```python
from build123d import *

# Parameters (mm, degrees)
F0_W            = 31.75
F0_H            = 6.35
F0_W_2          = 12.7
F0_H_2          = 101.6
F1_DEPTH        = 6.35
F2_DEPTH        = 76.2
F3_W            = 12.7
F3_H            = 68.58
F4_DEPTH        = 6.35
F5_W            = 12.7
F5_H            = 22.225
F6_DEPTH        = 6.35
F7_D            = 1.5875
F7_CSINK_D      = 3.175
F7_CSINK_ANGLE  = 90
F8_R            = 6.34999
F10_D           = 3.175
F12_D           = 3.175
F12_CSINK_D     = 6.35
F12_CSINK_ANGLE = 90
F13_R           = 1.5875
F14_DEPTH       = 12.7


# Not quite as in the source:
# - a fillet or chamfer is up to 0.001 mm smaller than in the source, because OpenCascade refuses the exact size


with BuildPart() as f1:
    # F0 (on Front) → F1 (new body)
    with BuildSketch(Plane.XZ):
        with Locations((-22.225, 174.625)):
            Rectangle(F0_W, F0_H)
        with Locations((22.225, 174.625)):
            Rectangle(F0_W, F0_H)
        with Locations((-22.225, 3.175)):
            Rectangle(F0_W, F0_H)
        with Locations((22.225, 3.175)):
            Rectangle(F0_W, F0_H)
        Polygon((-6.35, 171.45), (-38.1, 171.45), (-38.1, 108.712), (-31.75, 108.712), (-31.75, 69.088), (-38.1, 69.088), (-38.1, 6.35), (-6.35, 6.35), (-6.35, 22.225), (6.35, 22.225), (6.35, 6.35), (38.1, 6.35), (38.1, 69.088), (31.75, 69.088), (31.75, 108.712), (38.1, 108.712), (38.1, 171.45), (6.35, 171.45), (6.35, 161.925), (-6.35, 161.925), align=None)
        with Locations((0, 92.075)):
            Rectangle(F0_W_2, F0_H_2, mode=Mode.SUBTRACT)
    extrude(amount=F1_DEPTH)

    # F0 (on Front) → F2 (join)
    with BuildSketch(Plane.XZ):
        with Locations((-22.225, 174.625)):
            Rectangle(F0_W, F0_H)
        with Locations((22.225, 174.625)):
            Rectangle(F0_W, F0_H)
        with Locations((-22.225, 3.175)):
            Rectangle(F0_W, F0_H)
        with Locations((22.225, 3.175)):
            Rectangle(F0_W, F0_H)
        with Locations((0, 3.175)):
            Rectangle(F0_W_2, F0_H)
        with Locations((0, 174.625)):
            Rectangle(F0_W_2, F0_H)
    extrude(amount=F2_DEPTH)

    # F3 (on face) → F4 (cut, through all)
    with BuildSketch(Plane.XY.offset(177.8)):
        with Locations((0, -34.29)):
            Rectangle(F3_W, F3_H)
    extrude(amount=-F4_DEPTH, mode=Mode.SUBTRACT)

    # F5 (on face) → F6 (cut, through all)
    with BuildSketch(Plane(origin=(0, 0, 0), x_dir=(1, 0, 0), z_dir=(0, 0, -1))):
        with Locations((0, 11.1125)):
            Rectangle(F5_W, F5_H)
    extrude(amount=-F6_DEPTH, mode=Mode.SUBTRACT)

    # F7 (through all)
    with Locations(Plane(origin=(0, 0, 0), x_dir=(1, 0, 0), z_dir=(0, 1, 0))):
        with Locations((-3.175, -158.75), (3.175, -158.75)):
            CounterSinkHole(F7_D / 2, F7_CSINK_D / 2, counter_sink_angle=F7_CSINK_ANGLE)

    # F8 (radius 6.35 in the source; OpenCascade refuses exactly that, so slightly less here)
    f8_edges = [f1.edges().sort_by_distance(p)[0] for p in [
        (-6.35, -3.175, 22.225),
        (6.35, -3.175, 22.225),
        (-6.35, -3.175, 161.925),
        (6.35, -3.175, 161.925),
        (-6.35, -68.58, 174.625),
        (6.35, -68.58, 174.625),
        (6.35, -22.225, 3.175),
        (-6.35, -22.225, 3.175),
        (-6.35, -3.175, 41.275),
        (6.35, -3.175, 41.275),
        (-6.35, -3.175, 142.875),
        (6.35, -3.175, 142.875),
    ]]
    fillet(f8_edges, radius=F8_R)

    # F10 (through all)
    with Locations(Plane.YZ.offset(38.1)):
        with Locations((-3.175, 88.9)):
            Hole(F10_D / 2)

    # F12 (through all)
    with Locations(Plane(origin=(0, 0, 0), x_dir=(1, 0, 0), z_dir=(0, 0, -1))):
        with Locations((0, 34.925)):
            CounterSinkHole(F12_D / 2, F12_CSINK_D / 2, counter_sink_angle=F12_CSINK_ANGLE)

    # F13 (on Right) → F14 (cut, symmetric)
    with BuildSketch(Plane.YZ):
        with Locations((-55.5625, 174.625)):
            Circle(F13_R)
    extrude(amount=F14_DEPTH, both=True, mode=Mode.SUBTRACT)


solid = f1.part
```
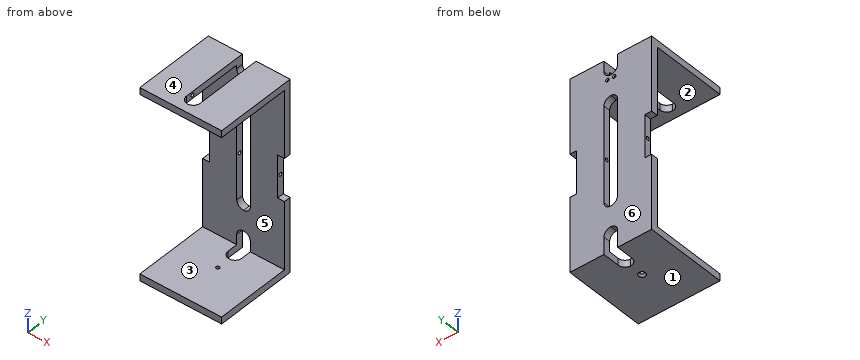
Geometry check sheet. Reference: the model listing, model coordinates, mm. Face numbers are marked on the shaded views. A direction names the side the tool comes from. Round coordinates to 2 decimals unless told otherwise and drop trailing zeros. Loops run counter-clockwise (first coordinate to the right, second up) from the corner with the lowest first, then second, coordinate; pieces in that order, holes last. Notation, with made-up numbers: (-16, -25.5) - (33, -25.5) arc R24 ccw to (33, 13.5) - close; hole circle Ø8 at (-9, -35). An arc over 180 degrees is marked (long way). Write each question's results on one line, items separated by ' | '. Start each with the question number.
Q1. Thickness scan on line 1 (X direction, y = -2.2, z = 158.75); line 2 (Z direction, x = 27, y = -46.5); line 3 (Y direction, x = -22.5, z = 88.9). Record the ranges inside material, lowest first. Write a range as [from, to].
Q2. Cross-section at C-C on y = -64. Enter the section's corners in (x, z), and give its area (3 significant figures).
Q3. Cross-section at B-B on z = 97.5. Enter the section's corners in (x, y).
Q4. Gauge pin test, flat ends, axial feed: P1, Ø3, axis at x = 0, y = -34.925, coming from the +Z side; P2, Ø1.9, axis at y = -2.5, z = 96.5, coming from the +X side; P3, Ø1.5, axis at x = -6, y = -45.5, coming from the +Z side; P4, Ø5, axis at y = -1.5, z = 93.5, coming from the -X side. Record the tip position at first contact, or that the pin passes through.
Q5. Release check for a two-part mould opening along Z. For the marked faces 1, 2, 3 and 4 record: +Z half, -Z half, draft (parallel to the pull), parting line (faces both ways), or undercut.
Q6. Access from +Z, -Z, +X, -X, +Y, -Y to the whole of each face (thin tool, end or side, straight path). Record for the marked faces 5 and 6.
Q7. Cross-section at D-D on z = 27. Enter the section's corners in (x, y).
Answers below:
1) line 1: x = [-38.1, -3.97], [-2.38, 2.38], [3.97, 38.1] | line 2: z = [0, 6.35], [171.45, 177.8] | line 3: y = [-6.35, -4.76], [-1.59, 0]
2) outline: (-38.1, 0) - (38.1, 0) - (38.1, 6.35) - (-38.1, 6.35) - close; (-38.1, 171.45) - (-6.1, 171.45) - (-6.1, 177.8) - (-38.1, 177.8) - close; (6.1, 171.45) - (38.1, 171.45) - (38.1, 177.8) - (6.1, 177.8) - close | area: 890 mm²
3) outline: (-31.75, -6.35) - (-6.35, -6.35) - (-6.35, 0) - (-31.75, 0) - close; (6.35, -6.35) - (31.75, -6.35) - (31.75, 0) - (6.35, 0) - close
4) P1: passes through | P2: stops at x = 31.75 | P3: stops at z = 177.8 | P4: stops at x = -31.75
5) face 1: -Z half | face 2: undercut | face 3: undercut | face 4: +Z half
6) face 5: +X, -X, -Y | face 6: +Z, -Z, +X, -X, +Y
7) outline: (-38.1, -6.35) - (38.1, -6.35) - (38.1, 0) - (-38.1, 0) - close
